Input: dimensioned drawing with shaded views. Units: mm. Origin: part minimum x, y, z. A direction names the side the tool comes from. Give positions to 0.01 mm unless a question says otherwise; leave off trailing zeros. Write each loop counter-clockwise with the first axis right and the second up, starting at its lowest first coordinate (ties: lowest second). Pieces come first, ordered by that corner, then holes. Notation, with made-up numbers: (-15, 86.25) -> (26, 86.25) arc R18 cw to (26, 94.25) -> close; hole circle Ø9 at (45.5, 25.25). An arc over 180 degrees is marked (long way). Answer in a Markdown table with one row per item. Add a question column.
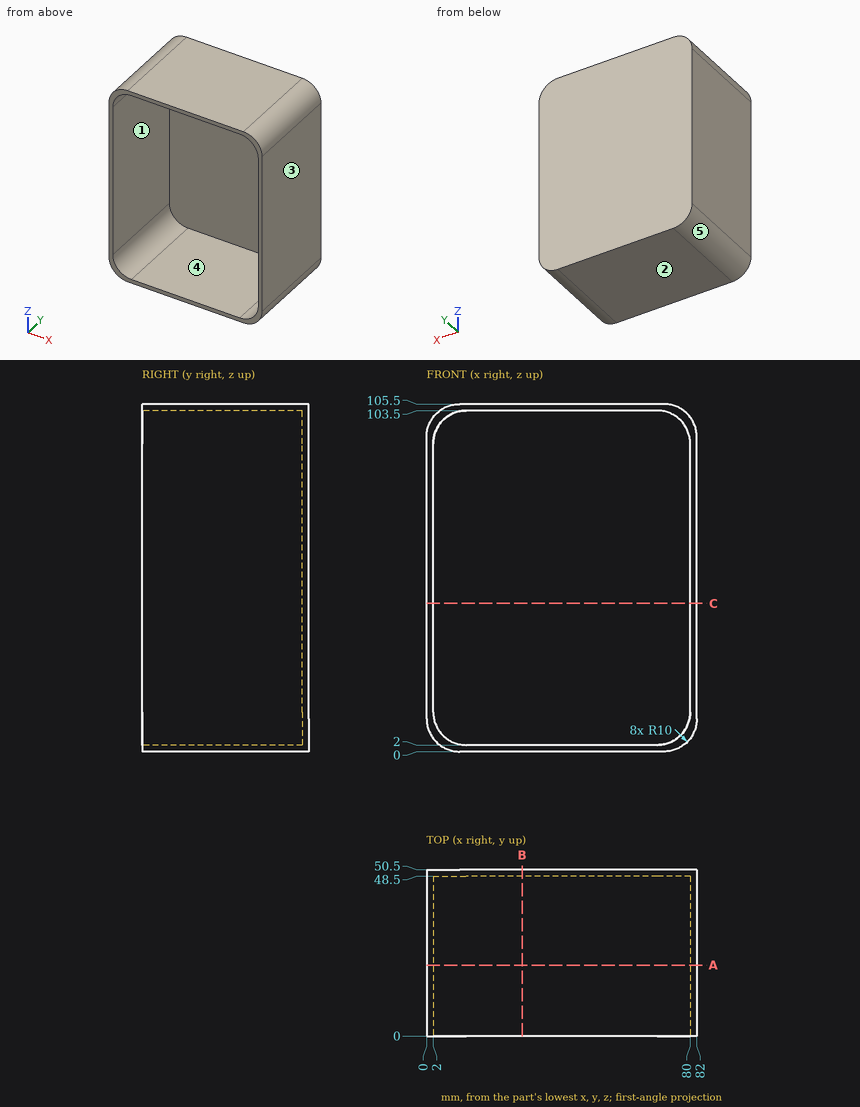
Q1. Section C-C on z = 45. Return loops of the section in (x, y).
Q2. Section A-A on y = 21.5. Return loops of the section in (x, z), and give its area (3 significant figures).
Q3. Line query: probe 1 along X at (y, z) = (39.5, 37); probe 2 along Z at (x, y) = (53, 22.5); probe 3 along Y at (x, z) = (50.5, 70.5). Output: solid intervals per line, ascending. Write a range as from..to.
Q4. Pull-direction query (Z, two-part tool) for the marked faces 1, 2 and 3; classes: +Z half, -Z half, draft (parallel to the pull), parting line (faces both ways), or undercut.
Q5. Contact query for a flat-ended pin moving along its axis: pin 1 Ø6 at (y, z) = (42, 72) entering from -X. Output: stop coordinate, or through.
Q6. Access query for the marked faces 4 and 5. Directions: +Z, -Z, +X, -X, +Y, -Y. A direction counts if a zero-diameter tool reaches every point of the face in a straight line with its end or side. Return the directions, or none.
Q7. Section B-B on x = 29. Return loops of the section in (y, z), and give its area (3 significant figures).
Checks:
| question | item | result |
|---|---|---|
| 1 | outline | (0, 0) -> (2, 0) -> (2, 48.5) -> (80, 48.5) -> (80, 0) -> (82, 0) -> (82, 50.5) -> (0, 50.5) -> close |
| 2 | outline | (0, 10) arc R10 ccw to (10, 0) -> (72, 0) arc R10 ccw to (82, 10) -> (82, 95.5) arc R10 ccw to (72, 105.5) -> (10, 105.5) arc R10 ccw to (0, 95.5) -> close; hole (2, 12) arc R10 ccw to (12, 2) -> (70, 2) arc R10 ccw to (80, 12) -> (80, 93.5) arc R10 ccw to (70, 103.5) -> (12, 103.5) arc R10 ccw to (2, 93.5) -> close |
| 2 | area | 734 mm^2 |
| 3 | probe 1 | 0..2, 80..82 |
| 3 | probe 2 | 0..2, 103.5..105.5 |
| 3 | probe 3 | 48.5..50.5 |
| 4 | face 1 | undercut |
| 4 | face 2 | -Z half |
| 4 | face 3 | draft |
| 5 | pin 1 | x = 0 |
| 6 | face 4 | -Y |
| 6 | face 5 | -Z, -X, +Y, -Y |
| 7 | outline | (0, 0) -> (50.5, 0) -> (50.5, 105.5) -> (0, 105.5) -> (0, 103.5) -> (48.5, 103.5) -> (48.5, 2) -> (0, 2) -> close |
| 7 | area | 405 mm^2 |
